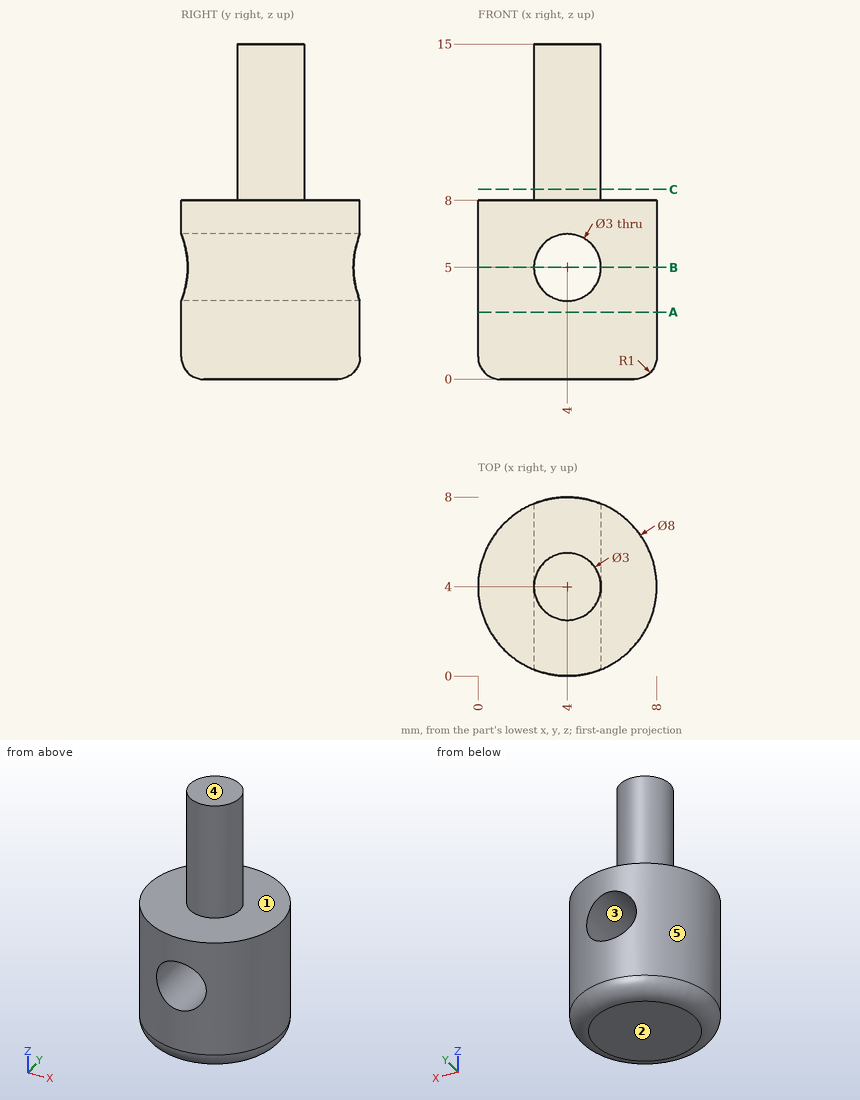
Study the drawing (mm; zero at the part's minimum x, y, z) and answer. A direction names the side the tool comes from. Coordinates: 2 decimals unless noted, no trailing zeros. Loops run counter-clockwise (first coordinate to the right, second up) from the corner with the lowest first, then second, coordinate; pieces in that order, holes last. Notation, with made-up numbers: (21, 24.25) -> (60, 24.25) arc R16 cw to (60, 48.25) -> close; hole circle Ø2 at (86, 50.25). An arc over 180 degrees is marked (long way). Answer as CSV lines item,"result".
1) The part is cut by section A-A (z = 3). Give the vertices of the cut face in (x, y), and give its area (3 significant figures).
A:
outline,"circle Ø8 at (4, 4)"
area,"50.3 mm²"
2) For the marked faces 1 and 2, determine the directions among +Z, -Z, +X, -X, +Y, -Y from which every point of the face is accessible in a straight line to the end or side of a thin tool.
A:
face 1,"+Z"
face 2,"-Z, +X, -X, +Y, -Y"
3) For a pull along X with two mould halves and no side action, classify the marked faces 3, 4 and 5 as released by +X, released by -X, zero draft, split by the parting line, or undercut.
A:
face 3,"undercut"
face 4,"zero draft"
face 5,"split by the parting line"
4) Flat-ended cylindrical pins translate along their axes: pin 1 (3 mm diameter, centred on y = 2, z = 5, fed in from -X); pin 2 (1.5 mm diameter, centred on x = 5, z = 10, fed in from +Y); pin 3 (3 mm diameter, centred on x = 1.5, z = 11, fed in from +Y). Find the tip coordinate at first contact, or state that the pin passes through.
A:
pin 1,"stops at x = 0.03"
pin 2,"stops at y = 5.48"
pin 3,"stops at y = 5.12"
5) The part is cut by section C-C (z = 8.5). Give the vertices of the cut face in (x, y).
A:
outline,"circle Ø3 at (4, 4)"
6) Straight lines are drawn through the part: probe 1 along X at (y, z) = (6.5, 5); probe 2 along X at (y, z) = (4.5, 5); probe 3 along Z at (x, y) = (4.25, 1.5). For each, find the intervals that lie inside material, in ascending order.
A:
probe 1,"x = 0.88 to 2.5, 5.5 to 7.12"
probe 2,"x = 0.03 to 2.5, 5.5 to 7.97"
probe 3,"z = 0 to 3.52, 6.48 to 8"
7) The part is cut by section B-B (z = 5). Give the vertices of the cut face in (x, y), and give its area (3 significant figures).
A:
outline,"(2.5, 0.29) -> (2.5, 7.71) arc R4 ccw to start; (5.5, 0.29) arc R4 ccw to (5.5, 7.71) -> close"
area,"26.8 mm²"
